from build123d import *

# Parameters (mm, degrees)
F1_DEPTH = 11.43
F2_R     = 1.7145
F3_DEPTH = 10.16
F4_W     = 0.4064
F4_H     = 5.1579866558
F5_DEPTH = 9.652
F6_SIZE  = 1.27
F7_R     = 2.54


with BuildPart() as f1:
    # F0 (on Top) → F1 (new body)
    with BuildSketch(Plane.XY):
        with BuildLine():
            ThreePointArc((-0.60325, 5.0440548607), (-3.372083184, -3.7994019266), (5.08, 0))
            ThreePointArc((5.08, 0), (3.7994019266, 3.372083184), (0.60325, 5.0440548607))
            Line((0.60325, 5.0440548607), (0.60325, 3.6805351715))
            Line((0.60325, 3.6805351715), (-0.60325, 3.6805351715))
            Line((-0.60325, 3.6805351715), (-0.60325, 5.0440548607))
        make_face()
        with BuildLine():
            Line((0.60325, 3.6805351715), (0.60325, 5.0440548607))
            ThreePointArc((0.60325, 5.0440548607), (0, 5.08), (-0.60325, 5.0440548607))
            Line((-0.60325, 5.0440548607), (-0.60325, 3.6805351715))
            Line((-0.60325, 3.6805351715), (0.60325, 3.6805351715))
        make_face()
        with BuildLine():
            ThreePointArc((-0.60325, 5.0440548607), (0, 5.08), (0.60325, 5.0440548607))
            Line((0.60325, 5.0440548607), (0.60325, 6.4794648285))
            Line((0.60325, 6.4794648285), (-0.60325, 6.4794648285))
            Line((-0.60325, 6.4794648285), (-0.60325, 5.0440548607))
        make_face()
    extrude(amount=-F1_DEPTH)

    # F2 (on face) → F3 (cut)
    with BuildSketch(Plane.XY):
        Circle(F2_R)
    extrude(amount=-F3_DEPTH, mode=Mode.SUBTRACT)

    # F4 (on Top) → F5 (join)
    with BuildSketch(Plane.XY):
        Rectangle(F4_W, F4_H)
    extrude(amount=-F5_DEPTH)

    # F6
    f6_edges = [f1.edges().sort_by_distance(p)[0] for p in [
        (0, -5.08, -11.43),
    ]]
    chamfer(f6_edges, length=F6_SIZE)

    # F7
    f7_edges = [f1.edges().sort_by_distance(p)[0] for p in [
        (0, 6.479465, -11.43),
    ]]
    fillet(f7_edges, radius=F7_R)


solid = f1.part
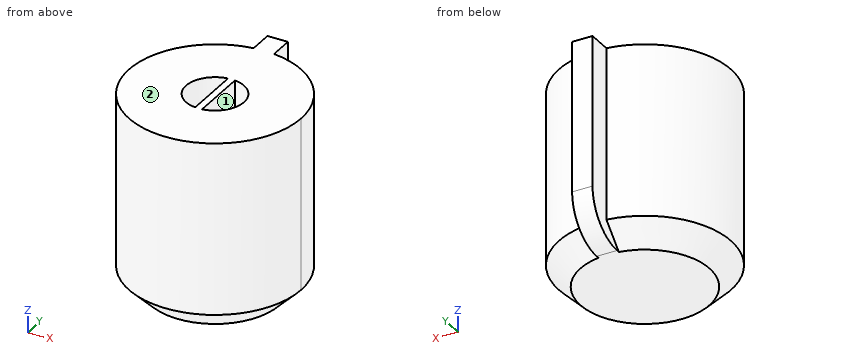
Could you check a few things on this model? Use its own coordinates, in mm. Face numbers are marked on the shaded views. Coordinates: 2 decimals unless noted, no trailing zeros. Write each loop counter-clockwise with the first axis right and the second up, starting at its lowest first coordinate (ties: lowest second). Pieces come first, ordered by that corner, then holes. Notation, with made-up numbers: (-1.5, 21.5) - (31.5, 21.5) arc R27 ccw to (31.5, 44.5) - close; hole circle Ø8 at (58, 1.5). An arc over 180 degrees is marked (long way). Write item = value, one per line.
1) We'd pull the mould along X, two halves only. Please class the marked faces 1 and 2: +X half, -X half, draft (parallel to the pull), parting line (faces both ways), or undercut.
Result set:
face_1 = undercut
face_2 = draft
2) Suppose I cut it at C-C on y = 5.5. Please give me the cut outline in (x, z).
Result set:
outline = (-0.6, -10.89) - (0.6, -10.89) - (0.6, 0) - (-0.6, 0) - close
3) Suppose I cut it at A-A on x = 0. Please give me the cut outline in (y, z).
Result set:
outline = (-5.08, -10.16) - (-3.81, -11.43) - (3.94, -11.43) arc R2.54 ccw to (6.48, -8.89) - (6.48, 0) - (-5.08, 0) - close; hole (-1.71, -10.16) - (1.71, -10.16) - (1.71, -9.65) - (-1.71, -9.65) - close
4) Please list where these lines run through material, in increasing order: line 1 (X direction, y = 0, z = -7.5); line 2 (Y direction, x = 0.5, z = -3.75); line 3 (Y direction, x = -0.25, z = -2.75). Write a range as [from, to].
Result set:
line_1 = [-5.08, -1.71], [-0.2, 0.2], [1.71, 5.08]
line_2 = [-5.06, -1.64], [1.64, 6.48]
line_3 = [-5.07, -1.7], [1.7, 6.48]
5) Will these pins go through, and if not, where does the flat tip stop? pin 1 Ø3 at (y, z) = (4.5, -8.5) entering from -X; pin 2 Ø1 at (x, z) = (-3.5, -4) entering from +Y.
Result set:
pin_1 = -4.1
pin_2 = 4.1
6) Suppose I cut it at B-B on z = -8. Please give me the cut outline in (x, y), plus the area to 3 significant figures.
Result set:
outline = (-0.6, 5.04) arc R5.08 ccw (long way) to (0.6, 5.04) - (0.6, 6.48) - (-0.6, 6.48) - close; hole (-0.2, -1.7) - (-0.2, 1.7) arc R1.71 ccw to start; hole (0.2, -1.7) arc R1.71 ccw to (0.2, 1.7) - close
area = 74.9 mm2
